```python
from build123d import *

# Parameters (mm, degrees)
BOSS_EXTRUDE1_DEPTH = 546.1
SKETCH2_R           = 49.5046
SKETCH2_R_2         = 47.6885
BOSS_EXTRUDE2_DEPTH = 203.2
BOSS_EXTRUDE3_START = 101.6
SKETCH3_R           = 49.5046
SKETCH3_R_2         = 47.6885
BOSS_EXTRUDE3_DEPTH = 101.6


with BuildPart() as part:
    # Sketch1 → Boss-Extrude1 (new body)
    with BuildSketch(Plane.XY):
        with BuildLine():
            Line((-49.5046, 0), (-47.6885, 0))
            ThreePointArc((-47.6885, 0), (0, -47.6885), (47.6885, 0))
            Line((47.6885, 0), (49.5046, 0))
            ThreePointArc((49.5046, 0), (0, -49.5046), (-49.5046, 0))
        make_face()
    extrude(amount=BOSS_EXTRUDE1_DEPTH)

    # Sketch2 → Boss-Extrude2 (add)
    with BuildSketch(Plane.XY.offset(546.1)):
        Circle(SKETCH2_R)
        Circle(SKETCH2_R_2, mode=Mode.SUBTRACT)
    extrude(amount=BOSS_EXTRUDE2_DEPTH)

    # Sketch3 → Boss-Extrude3 (add)
    with BuildSketch(Plane(origin=(0, 0, 0), x_dir=(-1, 0, 0), z_dir=(0, 0, -1)).offset(BOSS_EXTRUDE3_START)):
        Circle(SKETCH3_R)
        Circle(SKETCH3_R_2, mode=Mode.SUBTRACT)
    extrude(amount=-BOSS_EXTRUDE3_DEPTH)


solid = part.part
```
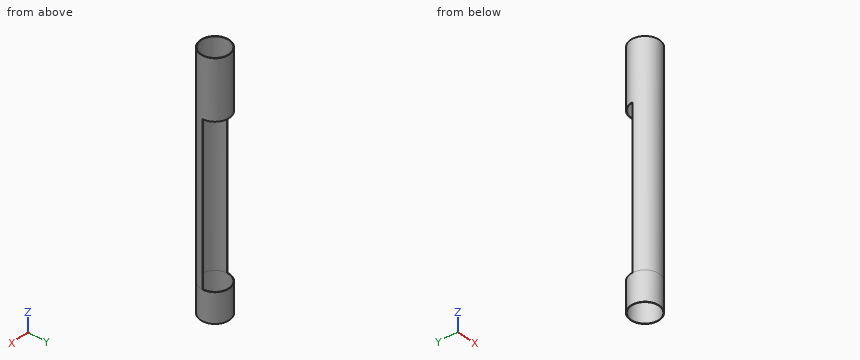
Check sheet for the modelled part. Datum: model origin and axes. Units: mm. Give positions to 0.01 mm unless a question says otherwise; leave off trailing zeros. Write each loop counter-clockwise with the first axis right and the second up, starting at its lowest first coordinate (ties: lowest second). Pieces come first, ordered by that corner, then holes.
Item 1: Scan lines: L1, parallel to Y at x = 0, z = -33; L2, parallel to X at y = -2.5, z = 300.5. Record each from-to range of solid material in increasing order.
Item 2: Cross-section at A-A (x = 0). Enter the section's corners in (y, z), and give its area (3 significant figures).
Item 3: Gauge pin test, flat ends, axial feed: pin 1 (0.9 mm diameter, centred on x = 48.5, z = 345.5, fed in from +Y); pin 2 (12 mm diameter, centred on x = 2.5, z = 500.5, fed in from +Y); pin 3 (1 mm diameter, centred on x = 18.5, z = 541.5, fed in from +Y). Record the tip position at first contact, or that the pin passes through.
Item 4: Cross-section at C-C (y = 39.5). Enter the section's corners in (x, z).
Item 5: Cross-section at B-B (y = -33). Enter the section's corners in (x, z).
Item 6: Cross-section at D-D (z = 209). Enter the section's corners in (x, y), and give its area (3 significant figures).
Report:
1. L1: y = -49.5 to -47.69, 47.69 to 49.5
1. L2: x = -49.44 to -47.62, 47.62 to 49.44
2. outline: (-49.5, -101.6) - (-47.69, -101.6) - (-47.69, 749.3) - (-49.5, 749.3) - close; (47.69, -101.6) - (49.5, -101.6) - (49.5, 0) - (47.69, 0) - close; (47.69, 546.1) - (49.5, 546.1) - (49.5, 749.3) - (47.69, 749.3) - close
2. area: 2,100 mm2
3. pin 1: stops at y = 0
3. pin 2: stops at y = -46.92
3. pin 3: stops at y = -43.74
4. outline: (-29.84, -101.6) - (-26.72, -101.6) - (-26.72, 0) - (-29.84, 0) - close; (-29.84, 546.1) - (-26.72, 546.1) - (-26.72, 749.3) - (-29.84, 749.3) - close; (26.72, -101.6) - (29.84, -101.6) - (29.84, 0) - (26.72, 0) - close; (26.72, 546.1) - (29.84, 546.1) - (29.84, 749.3) - (26.72, 749.3) - close
5. outline: (-36.9, -101.6) - (-34.43, -101.6) - (-34.43, 749.3) - (-36.9, 749.3) - close; (34.43, -101.6) - (36.9, -101.6) - (36.9, 749.3) - (34.43, 749.3) - close
6. outline: (-49.5, 0) arc R49.5 ccw to (49.5, 0) - (47.69, 0) arc R47.69 cw to (-47.69, 0) - close
6. area: 277 mm2
